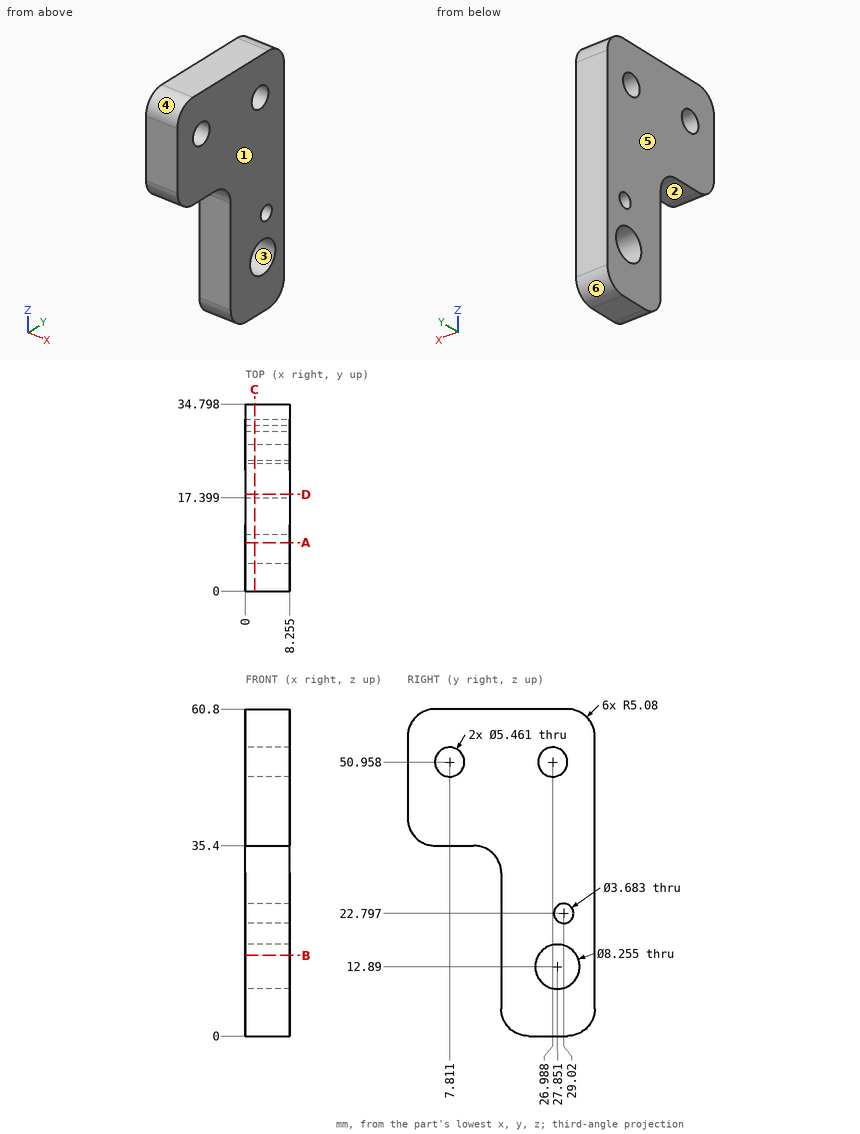
Drawing for the job (mm, zero at the part's lowest x, y, z). A direction names the side the tool comes from. Give positions to 0.01 mm unless a question says otherwise; leave off trailing zeros. Loops run counter-clockwise (first coordinate to the right, second up) from the corner with the lowest first, then second, coordinate; pieces in that order, holes last.
1) Probe line 1 along Y through (x, z) = (1.25, 51); line 2 along Z through (x, y) = (3, 25) (1 decimal); line 3 along Z through (x, y) = (2.5, 27). List the from-to ranges inside material, lowest first.
Values follow:
line 1: y = 0 to 5.08, 10.54 to 24.26, 29.72 to 34.8
line 2: z = 0 to 9.9, 15.9 to 49.1, 52.8 to 60.8
line 3: z = 0 to 8.85, 16.93 to 48.23, 53.69 to 60.8
2) Band-saw the part on B-B on z = 15. List the corners of the cut face in (x, y) (1 decimal).
Values follow:
outline: (0, 17.4) - (8.3, 17.4) - (8.3, 24.3) - (0, 24.3) - close; (0, 31.4) - (8.3, 31.4) - (8.3, 34.8) - (0, 34.8) - close
3) 3-axis set-ups, long thin cutter, end or side, ignore diameter. For the marked faces 1 and 2: which of +Z, -Z, +X, -X, +Y, -Y reach the whole face in a straight line?
Values follow:
face 1: +Z, -Z, +X, +Y, -Y
face 2: -Z, +X, -X, -Y
4) Band-saw the part on C-C on x = 1.75. List the corners of the cut face in (y, z) (1 decimal), then the cut area to 3 significant figures.
Values follow:
outline: (0, 40.5) arc R5.1 ccw to (5.1, 35.4) - (12.3, 35.4) arc R5.1 cw to (17.4, 30.3) - (17.4, 5.1) arc R5.1 ccw to (22.5, 0) - (29.7, 0) arc R5.1 ccw to (34.8, 5.1) - (34.8, 55.7) arc R5.1 ccw to (29.7, 60.8) - (5.1, 60.8) arc R5.1 ccw to (0, 55.7) - close; hole circle Ø5.5 at (7.8, 51); hole circle Ø8.3 at (27.9, 12.9); hole circle Ø5.5 at (27, 51); hole circle Ø3.7 at (29, 22.8)
area: 1,370 mm2
5) Band-saw the part on A-A on y = 9. List the corners of the cut face in (x, z) (1 decimal), then the cut area to 3 significant figures.
Values follow:
outline: (0, 35.4) - (8.3, 35.4) - (8.3, 48.5) - (0, 48.5) - close; (0, 53.4) - (8.3, 53.4) - (8.3, 60.8) - (0, 60.8) - close
area: 169 mm2
6) Band-saw the part on D-D on y = 18. List the corners of the cut face in (x, z) (1 decimal).
Values follow:
outline: (0, 2.7) - (8.3, 2.7) - (8.3, 60.8) - (0, 60.8) - close
7) Drop flat-ended pins along their axis: P1, Ø6, axis at y = 13.5, z = 9.5, coming from the -X side; P2, Ø3.5, axis at x = 2.5, y = 8, coming from the -Z side; P3, Ø4, axis at x = 4.5, z = 15.5, coming from the -Y side. Give the stop position or say it passes through.
Values follow:
P1: passes through
P2: stops at z = 35.4
P3: stops at y = 17.4
8) Two-plate mould, pull along Y, no slides. Class the marked faces 3, 4, 5 and 6: released by +Y, released by -Y, zero draft, split by the parting line, or undercut.
Values follow:
face 3: undercut
face 4: released by -Y
face 5: zero draft
face 6: released by +Y
